Autodesk Inventor part; units mm, degrees
ref_plane "YZ Plane" through (0, 0, 0) normal (1, 0, 0) x (0, 1, 0)
ref_plane "XZ Plane" through (0, 0, 0) normal (0, 1, 0) x (-1, 0, 0)
ref_plane "XY Plane" through (0, 0, 0) normal (0, 0, 1) x (1, 0, 0)
sketch "草圖1" plane through (0, 0, 0) normal (0, 1, 0) x (-1, 0, 0)
  circle A0 centre (0, 0) radius 15
  line L0 (0, 0) -> (15, 0)
  line L1 (0, 0) -> (7.5, -12.9904)
  line L2 (0, 0) -> (12.9904, -7.5)
  circle A1 centre (0, 0) radius 12.5
  circle A2 centre (0, 0) radius 5
  circle A3 centre (0, 0) radius 1.55
  point P0 (6.25, -10.8253)
  point P1 (2.5, -4.3301)
  point P2 (4.3301, -2.5)
  point P3 (10.8253, -6.25)
  dimension "d0" = 30
  dimension "d1" = 60
  dimension "d2" = 30
  dimension "d3" = 25
  dimension "d4" = 10
  dimension "d12" = 3.1
extrude "擠出1" add sketch "草圖1" along normal blind 3
extrude "擠出2" cut sketch "草圖1" along normal blind 3 contours L1 A2 L2 A1
pattern_circular "環形陣列1" count 6 over 360 about axis through (0, -10, 0) along (0, 1, 0) of "擠出2"
extrude "擠出3" cut sketch "草圖1" along normal blind 3 contours A3 L2 L0 | L0 L1 A3 | L1 L2 A3
fillet "圓角1" radius 1 24 edges at (-2.5, 1.5, -4.3301) (2.5, 1.5, -4.3301) (12.5, 1.5, 0) (0, 1.5, 12.5) (-4.3301, 1.5, 2.5) (-4.3301, 1.5, -2.5) (-6.25, 1.5, -10.8253) (0, 1.5, -12.5) (10.8253, 1.5, -6.25) (4.3301, 1.5, 2.5) (-2.5, 1.5, 4.3301) (-5, 1.5, 0) (6.25, 1.5, -10.8253) (0, 1.5, 5) (2.5, 1.5, 4.3301) (0, 1.5, -5) (-10.8253, 1.5, 6.25) (-6.25, 1.5, 10.8253) (6.25, 1.5, 10.8253) (10.8253, 1.5, 6.25) (-10.8253, 1.5, -6.25) (-12.5, 1.5, 0) (4.3301, 1.5, -2.5) (5, 1.5, 0)
properties material "MDF Medium Density Fiberboard"
Could you check a few things on this model? Use its own coordinates, in mm. Coordinates: 2 decimals unless noted, no trailing zeros. Order: outer loops, then holes, each group sorted by start corner. A loop starts at its lowest first (then second) coordinate and runs counter-clockwise, first axis right, second up. Notation, with made-up numbers: (56, 77) -> (64, 77) arc R6 ccw to (64, 83) -> close; hole circle Ø8 at (80.5, 47). An arc over 180 degrees is marked (long way). One line per question, with ' | ' between items.
Q1. Imagine slicing it at C-C on y = 0.7. State how many separate pieces and enclosed holes the cut face has, and give its area (3 significant figures).
Return value:
separate pieces: 1 | enclosed holes: 7 | area: 498 mm²
Q2. Imagine slicing it at D-D on x = 12. Please give me the cut outline in (y, z).
Return value:
outline: (0, -9) -> (3, -9) -> (3, -3.5) -> (0, -3.5) -> close; (0, -0.16) -> (3, -0.16) -> (3, 9) -> (0, 9) -> close
Q3. I'm going to push flat-ended pins straight in: P1, Ø1, axis at x = 5.5, y = 2, coming from the +Z side; P2, Ø2.5, axis at x = 0, z = 0, coming from the -Y side; P3, Ø0.9, axis at x = 9.5, y = 1.5, coming from the -Z side; P4, Ø4, axis at x = 3.5, z = -2.5, coming from the -Y side. Where does each tip first touch, or does it pass through?
Return value:
P1: z = 14.14 | P2: through | P3: z = -11.96 | P4: y = 0
Q4. Imagine slicing it at B-B on x = -8.75. Please give me the cut outline in (y, z), and give its area (3 significant figures).
Return value:
outline: (0, -12.18) -> (3, -12.18) -> (3, -8.93) -> (0, -8.93) -> close; (0, -5.05) -> (3, -5.05) -> (3, 0) -> (0, 0) -> close; (0, 5.05) -> (3, 5.05) -> (3, 12.18) -> (0, 12.18) -> close | area: 46.3 mm²
Q5. Imagine slicing it at A-A on z = -12. Please give me the cut outline in (x, y).
Return value:
outline: (-9, 0) -> (0.16, 0) -> (0.16, 3) -> (-9, 3) -> close; (3.5, 0) -> (9, 0) -> (9, 3) -> (3.5, 3) -> close
Q6. If I drill on L1, parallel to X at y = 0.3, z = 2.75; L2, parallel to X at y = 2.1, z = 6.25; L3, parallel to Z at x = -7, y = 1.85, over which ranges is the centre line in solid material (lowest first)?
Return value:
L1: -14.75 to -12.19, -4.87 to 14.75 | L2: -13.64 to -3.61, 0 to 3.61, 10.36 to 13.64 | L3: -13.27 to -10.34, -4.04 to 0, 4.04 to 13.27
